Geometry check sheet. Reference: the model listing, model coordinates, mm. A direction names the side the tool comes from. Round coordinates to 2 decimals unless told otherwise and drop trailing zeros. Order: outer loops, then holes, each group sorted by start corner. A loop starts at its lowest first (then second) coordinate and runs counter-clockwise, first axis right, second up.
(1) Material ranges on line 1 along X through (y, z) = (1.2, 18); line 2 along Z through (x, y) = (51, 26.5); line 3 along Y through (x, z) = (16, 22.25), recorded low to high.
(2) Set-up check for faces 1 (the face through (197, 4, 17)), 2 (the face through (197, 0, 15)): record each of +Z, -Z, +X, -X, +Y, -Y from which the full face is reachable in a straight line by a thin tool's end or side.
(3) Sectioned sample at C-C (x = 228.5). Record the boundary of the cut face in (y, z), plus the area to 3 significant figures.
(4) Sectioned sample at A-A (x = 150). Record the boundary of the cut face in (y, z), plus the area to 3 significant figures.
(5) Release check for a two-part mould opening along X. For faces 3 (the face through (197, 17, 4)), 4 (the face through (0, 6, 4)), 5 (the face through (154.214, 2.028, 17.447)) record: +X half, -X half, draft (parallel to the pull), parting line (faces both ways), or undercut.
(6) Go/stop test with flat-tipped pins: pin 1 (7.5 mm diameter, centred on x = 150, z = 18, fed in from +Y) (3 decimals); pin 2 (10 mm diameter, centred on x = 306, z = 7, fed in from +Y); pin 3 (3 mm diameter, centred on x = 70, y = 10.5, fed in from +Z); pin 4 (12 mm diameter, centred on y = 13, z = 5.5, fed in from +X). Record where each tip stops, or that it passes through.
(7) Sectioned sample at B-B (z = 18). Record the boundary of the cut face in (x, y), plus the area to 3 significant figures.
from build123d import *

# Parameters (mm, degrees)
ANGLE_IRON_25_X_25_X_4_1_DEPTH = 400
SKETCH12_R                     = 4.25
CUT_EXTRUDE1_DEPTH             = 10


with BuildPart() as part:
    # Sketch11 → Angle iron 25 X 25 X 4(1) (new body)
    with BuildSketch(Plane.YZ):
        with BuildLine():
            Line((0, 0), (0, 30))
            ThreePointArc((0, 30), (2.828427125, 28.828427125), (4, 26))
            Line((4, 26), (4, 7.5))
            ThreePointArc((4, 7.5), (5.025126266, 5.025126266), (7.5, 4))
            Line((7.5, 4), (26, 4))
            ThreePointArc((26, 4), (28.828427125, 2.828427125), (30, 0))
            Line((30, 0), (0, 0))
        make_face()
    extrude(amount=ANGLE_IRON_25_X_25_X_4_1_DEPTH)

    # Sketch12 → Cut-Extrude1 (cut)
    with BuildSketch(Plane(origin=(0, 4, 0), x_dir=(1, 0, 0), z_dir=(0, 1, 0))):
        with Locations(Location((50, -18, 0), (0, 0, 270))):
            Circle(SKETCH12_R)
        with Locations(Location((150, -18, 0), (0, 0, 270))):
            Circle(SKETCH12_R)
        with Locations(Location((250, -18, 0), (0, 0, 270))):
            Circle(SKETCH12_R)
    extrude(amount=-CUT_EXTRUDE1_DEPTH, mode=Mode.SUBTRACT)


solid = part.part
Answer below:
1. line 1: x = 0 to 45.75, 54.25 to 145.75, 154.25 to 245.75, 254.25 to 400
1. line 2: z = 0 to 3.97
1. line 3: y = 0 to 4
2. face 1: +Z, +X, -X, +Y
2. face 2: +Z, -Z, +X, -X, -Y
3. outline: (0, 0) - (30, 0) arc R4 ccw to (26, 4) - (7.5, 4) arc R3.5 cw to (4, 7.5) - (4, 26) arc R4 ccw to (0, 30) - close
3. area: 220 mm2
4. outline: (0, 0) - (30, 0) arc R4 ccw to (26, 4) - (7.5, 4) arc R3.5 cw to (4, 7.5) - (4, 13.75) - (0, 13.75) - close; (0, 22.25) - (4, 22.25) - (4, 26) arc R4 ccw to (0, 30) - close
4. area: 186 mm2
5. face 3: draft
5. face 4: -X half
5. face 5: undercut
6. pin 1: passes through
6. pin 2: stops at y = 29.46
6. pin 3: stops at z = 4
6. pin 4: stops at x = 400
7. outline: (0, 0) - (45.75, 0) - (45.75, 4) - (0, 4) - close; (54.25, 0) - (145.75, 0) - (145.75, 4) - (54.25, 4) - close; (154.25, 0) - (245.75, 0) - (245.75, 4) - (154.25, 4) - close; (254.25, 0) - (400, 0) - (400, 4) - (254.25, 4) - close
7. area: 1,500 mm2
